Could you check a few things on this model? Use its own coordinates, in mm. A direction names the side the tool comes from. Give positions to 0.01 mm unless a question says otherwise; leave off trailing zeros. Order: outer loops, then holes, each group sorted by start corner. A loop starts at its lowest first (then second) coordinate and runs counter-clockwise, first axis right, second up.
from build123d import *

# Parameters (mm, degrees)
BOX_W           = 15
BOX_H           = 83
BOX_DEPTH       = 3
FILLET_R        = 5
SKETCH_W        = 6
SKETCH_H        = 83
PAD_DEPTH       = 2
SKETCH001_W     = 81
SKETCH001_H     = 0.2
POCKET_DEPTH    = 5
CHAMFER_SIZE    = 1.5
SKETCH002_R     = 2.5
POCKET001_DEPTH = 5


with BuildPart() as part:
    # Box → Box (new body)
    with BuildSketch(Plane.XY):
        with Locations((7.5, 41.5)):
            Rectangle(BOX_W, BOX_H)
    extrude(amount=BOX_DEPTH)

    # Fillet
    fillet_edges = [part.edges().sort_by_distance(p)[0] for p in [
        (0, 0, 1.5),
        (0, 83, 1.5),
    ]]
    fillet(fillet_edges, radius=FILLET_R)

    # Sketch (on Face2 of BaseFeature) → Pad (new body)
    with BuildSketch(Plane.XY.offset(3)):
        with Locations((12, 41.5)):
            Rectangle(SKETCH_W, SKETCH_H)
    extrude(amount=PAD_DEPTH)

    # Sketch001 (on Face10 of Pad) → Pocket (cut)
    with BuildSketch(Plane.YZ.offset(15)):
        with Locations((41.5, 2.5)):
            Rectangle(SKETCH001_W, SKETCH001_H)
    extrude(amount=-POCKET_DEPTH, mode=Mode.SUBTRACT)

    # Chamfer
    chamfer_edges = [part.edges().sort_by_distance(p)[0] for p in [
        (9, 41.5, 3),
    ]]
    chamfer(chamfer_edges, length=CHAMFER_SIZE)

    # Sketch002 (on Face5 of Chamfer) → Pocket001 (cut)
    with BuildSketch(Plane.XY.offset(3)):
        with Locations((3.75, 41.5)):
            Circle(SKETCH002_R)
    extrude(amount=-POCKET001_DEPTH, mode=Mode.SUBTRACT)


solid = part.part
Item 1: For faces 1 (the flat face through (13, 41, 2.4)), 2 (the flat face through (15, 41, 2)), which set-ups out of +Z, -Z, +X, -X, +Y, -Y let a thin tool reach every point of the face, with its end or its side?
Findings:
face 1: +X
face 2: +Z, -Z, +X, +Y, -Y
Item 2: Imagine slicing it at A-A on y = 41.5. List the corners of the cut face in (x, z) for me, then the cut area to 3 significant figures.
Findings:
outline: (0, 0) - (1.25, 0) - (1.25, 3) - (0, 3) - close; (6.25, 0) - (15, 0) - (15, 2.4) - (10, 2.4) - (10, 2.6) - (15, 2.6) - (15, 5) - (9, 5) - (9, 4.5) - (7.5, 3) - (6.25, 3) - close
area: 42.1 mm2
Item 3: Imagine slicing it at C-C on z = 1.65. List the corners of the cut face in (x, y) for me.
Findings:
outline: (0, 5) arc R5 ccw to (5, 0) - (15, 0) - (15, 83) - (5, 83) arc R5 ccw to (0, 78) - close; hole circle Ø5 at (3.75, 41.5)
Item 4: Please list where these lines run through material, in increasing order: line 1 along Z through (x, y) = (13, 35); line 2 along Y through (x, z) = (11.5, 2.5); line 3 along Y through (x, z) = (3.75, 2.1).
Findings:
line 1: z = 0 to 2.4, 2.6 to 5
line 2: y = 0 to 1, 82 to 83
line 3: y = 0.16 to 39, 44 to 82.84
Item 5: Imagine slicing it at B-B on x = 10.75. List the corners of the cut face in (y, z) for me, then the cut area to 3 significant figures.
Findings:
outline: (0, 0) - (83, 0) - (83, 5) - (0, 5) - close; hole (1, 2.4) - (82, 2.4) - (82, 2.6) - (1, 2.6) - close
area: 399 mm2
Item 6: For pin 1 (4 mm diameter, centred on x = 3.75, y = 41.5, fed in from -Z); pin 2 (8.5 mm diameter, centred on x = 4.5, y = 48.5, fed in from +Z), each with a flat end and sliding along its axis, tell me the tip position at first contact or that it passes through.
Findings:
pin 1: passes through
pin 2: stops at z = 4.25
Item 7: Imagine slicing it at D-D on x = 3.5. List the corners of the cut face in (y, z) for me.
Findings:
outline: (0.23, 0) - (39.01, 0) - (39.01, 3) - (0.23, 3) - close; (43.99, 0) - (82.77, 0) - (82.77, 3) - (43.99, 3) - close
Item 8: We'd pull the mould along X, two halves only. Please class faces 3 (the flat face through (1, 42, 3)), 4 (the cylindrical face through (3.21, 39.06, 1.52)), 5 (the cylindrical face through (1, 81, 2)): +X half, -X half, draft (parallel to the pull), parting line (faces both ways), or undercut.
Findings:
face 3: draft
face 4: undercut
face 5: -X half
